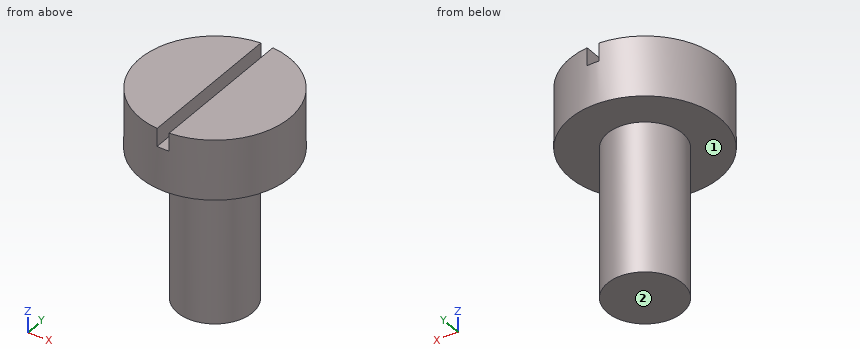
```python
from build123d import *

# Parameters (mm, degrees)
EXTRUDE_1_DEPTH      = 5
EXTRUDE_1_DEPTH_BACK = 5
SKETCH_1_R           = 2.5
SKETCH_2_R           = 5
EXTRUDE_2_DEPTH      = 4
SKETCH_3_W           = 0.8
SKETCH_3_H           = 11.021006482
CUT_EXTRUDE_1_DEPTH  = 1.2


with BuildPart() as part:
    # Sketch 1 → Extrude 1 (new, two sides: drawn at the far end of the back side and taken through both)
    with BuildSketch(Plane.XY.offset(-EXTRUDE_1_DEPTH_BACK)):
        Circle(SKETCH_1_R)
    extrude(amount=EXTRUDE_1_DEPTH + EXTRUDE_1_DEPTH_BACK)

    # Sketch 2 → Extrude 2 (add)
    with BuildSketch(Plane.XY.offset(5)):
        with Locations(Location((0, 0, 0), (0, 0, 94.588565736))):
            Circle(SKETCH_2_R)
    extrude(amount=EXTRUDE_2_DEPTH)

    # Sketch 3 → Cut-Extrude 1 (cut)
    with BuildSketch(Plane.XY.offset(9)):
        with Locations((0, 0.044379892)):
            Rectangle(SKETCH_3_W, SKETCH_3_H)
    extrude(amount=-CUT_EXTRUDE_1_DEPTH, mode=Mode.SUBTRACT)


solid = part.part
```
The model under review builds one solid part; all positions refer to its coordinate system, in mm. Face numbers are marked on the shaded views. A direction names the side the tool comes from. Round coordinates to 2 decimals unless told otherwise and drop trailing zeros. Loops run counter-clockwise (first coordinate to the right, second up) from the corner with the lowest first, then second, coordinate; pieces in that order, holes last. Notation, with made-up numbers: M -12,8.5 L 15,8.5 A30 ccw 15,44.5 Z; hole C 13.25,-38.5 d10. An arc over 180 degrees is marked long. Answer as a JSON object with one key per item and string values.
(1) Take a section at B-B on y = 0. Give the boundary of the cut face in (x, z), and give its area (3 significant figures).
Resolved:
{"outline": "M -5,5 L -2.5,5 L -2.5,-5 L 2.5,-5 L 2.5,5 L 5,5 L 5,9 L 0.4,9 L 0.4,7.8 L -0.4,7.8 L -0.4,9 L -5,9 Z", "area": "89.0 mm²"}
(2) Tool access review of the marked faces 1 and 2: name each direction out of +Z, -Z, +X, -X, +Y, -Y from which nothing blocks a thin tool from reaching the whole face with its end or side.
Resolved:
{"face 1": "-Z", "face 2": "-Z, +X, -X, +Y, -Y"}
(3) Clearance check with flat-ended pins moving along their axes: P1, Ø5, axis at x = -1, z = -1, coming from the +Y side; P2, Ø3, axis at y = 1, z = -2.5, coming from the -X side; P3, Ø5, axis at x = -0.5, z = 1.5, coming from the -Y side; P4, Ø1, axis at y = -3.5, z = 0, coming from the -X side. State where each tip first meets the part, or that it passes through.
Resolved:
{"P1": "y = 2.5", "P2": "x = -2.5", "P3": "y = -2.5", "P4": "through"}
(4) Take a section at D-D on z = -0.5. Give the boundary of the cut face in (x, y).
Resolved:
{"outline": "C 0,0 d5"}
(5) Take a section at C-C on x = 0. Give the boundary of the cut face in (y, z), and give its area (3 significant figures).
Resolved:
{"outline": "M -5,5 L -2.5,5 L -2.5,-5 L 2.5,-5 L 2.5,5 L 5,5 L 5,7.8 L -5,7.8 Z", "area": "78.0 mm²"}
(6) To check wall thickness, follow line 1 along Z through (x, y) = (0, 2); line 2 along Z through (x, y) = (2.25, -1.5); line 3 along Y through (x, z) = (0, -2.75). State the ranges of each line that lie inside material, in increasing order.
Resolved:
{"line 1": "-5 to 7.8", "line 2": "5 to 9", "line 3": "-2.5 to 2.5"}
